For this review, take the finished solid that the model builds, in its own axes (mm). A direction names the side the tool comes from. Coordinates: 2 decimals unless noted, no trailing zeros. Order: outer loops, then holes, each group sorted by start corner. A loop starts at its lowest first (then second) coordinate and runs counter-clockwise, first axis right, second up. Notation, with made-up numbers: (-8, 59) -> (40, 59) arc R17 ccw to (40, 63) -> close; hole circle Ø7 at (45.5, 12). An arc over 180 degrees is marked (long way). Return JSON: item names as keys, results as strings. Group by question number.
Item 1: Take a section at B-B (x = 0). Write out the cut boundary in (y, z), then the cut area to 3 significant figures.
Item 2: For line 1 along Z through (x, y) = (-9.75, -18); line 2 along Y through (x, z) = (0, 36.5); line 3 along Y through (x, z) = (-9.25, -17), list the stretches that pass through material, from the lowest coordinate up.
Item 3: Insertion check: pin 1 (3 mm diameter, centred on x = -8.5, y = -11.5, fed in from -Z); pin 2 (10 mm diameter, centred on y = 8, z = -17, fed in from +X); pin 3 (12 mm diameter, centred on x = -5, y = 11.5, fed in from -Z); pin 4 (5 mm diameter, centred on x = -2.5, z = 23.5, fed in from -Y). Each pin has a flat end and moves straight along its axis. Give the tip position at first contact, or say it passes through.
Item 4: Take a section at A-A (z = 25.5). Write out the cut boundary in (x, y), then the cut area to 3 significant figures.
Item 5: Take a section at D-D (x = 9). Write out the cut boundary in (y, z), then the cut area to 3 significant figures.
Item 6: Machinability: for faces 1 (the flat face through (0, 0, 8)), 2 (the flat face through (12.5, -1, 10)), 3 (the flat face through (-10, -12, 13)), 4 (the flat face through (-6.343, -3, -22)), 5 (the flat face through (-6.5, -12.6, 25.7)), which of the approach directions +Z, -Z, +X, -X, +Y, -Y give a long, thin tool a straight path to every point of the face, cutting with its end or side? Answer none if there is none.
Item 7: Draft analysis for pull direction Z (two halves, no side actions). For faces 6 (the cylindrical face through (-9.542, -30.497, 25.225)), 7 (the flat face through (6.657, -3, -22)), 8 (the cylindrical face through (-9.46, -19.08, 20.62)), state which applies: +Z half, -Z half, draft (parallel to the pull), parting line (faces both ways), or undercut.
Item 8: Take a section at C-C (y = 4.5). Write out the cut boundary in (x, z).
```python
from build123d import *

# Parameters (mm, degrees)
F0_W      = 25
F0_H      = 64
F1_DEPTH  = 6
F2_W      = 25
F2_H      = 6
F3_DEPTH  = 6
F5_DEPTH  = 6
F7_D      = 10
F7_DEPTH  = 13
F7_TIP    = 3.0043030951
F9_D      = 10
F9_DEPTH  = 13
F9_TIP    = 3.0043030951
F11_DEPTH = 12.4


with BuildPart() as f1:
    # F0 (on Front) → F1 (new body)
    with BuildSketch(Plane.XZ):
        Rectangle(F0_W, F0_H)
    extrude(amount=F1_DEPTH)

    # F2 (on face) → F3 (join)
    with BuildSketch(Plane.XY.offset(32)):
        with BuildLine():
            Line((-12.5, 12), (-12.5, 0))
            Line((-12.5, 0), (12.5, 0))
            Line((12.5, 0), (12.5, 12))
            ThreePointArc((12.5, 12), (0, 24.5), (-12.5, 12))
        make_face()
        with Locations((0, -3)):
            Rectangle(F2_W, F2_H)
    extrude(amount=F3_DEPTH)

    # F4 (on face) → F5 (join)
    with BuildSketch(Plane(origin=(-12.5, 0, 0), x_dir=(0, -1, 0), z_dir=(-1, 0, 0))):
        with BuildLine():
            Line((6, 38), (6, 13))
            Line((6, 13), (18, 13))
            ThreePointArc((18, 13), (30.5, 25.5), (18, 38))
            Line((18, 38), (6, 38))
        make_face()
    extrude(amount=-F5_DEPTH)

    # F7
    with Locations(Plane.XY.offset(38)):
        with Locations((0, 12)):
            Hole(F7_D / 2, depth=F7_DEPTH)
            with Locations((0, 0, -(F7_DEPTH + F7_TIP / 2))):  # 118° drill point
                Cone(0, F7_D / 2, F7_TIP, mode=Mode.SUBTRACT)

    # F9
    with Locations(Plane(origin=(-12.5, 0, 0), x_dir=(0, -1, 0), z_dir=(-1, 0, 0))):
        with Locations((18, 25.5)):
            Hole(F9_D / 2, depth=F9_DEPTH)
            with Locations((0, 0, -(F9_DEPTH + F9_TIP / 2))):  # 118° drill point
                Cone(0, F9_D / 2, F9_TIP, mode=Mode.SUBTRACT)

    # F10 (on face) → F11 (cut)
    with BuildSketch(Plane(origin=(0, 0, 0), x_dir=(-1, 0, 0), z_dir=(0, 1, 0))):
        with BuildLine():
            Line((-6.6569247283, -12), (-6.6569247283, -32))
            Line((-6.6569247283, -32), (6.3430752717, -32))
            Line((6.3430752717, -32), (6.3430752717, -12))
            ThreePointArc((6.3430752717, -12), (-0.1569247283, -5.5), (-6.6569247283, -12))
        make_face()
    extrude(amount=-F11_DEPTH, mode=Mode.SUBTRACT)


solid = f1.part
```
Findings below:
{
 "1": {"outline": "(-6, -5.5) -> (0, -5.5) -> (0, 32) -> (7, 32) -> (7, 38) -> (-6, 38) -> close; (17, 32) -> (24.5, 32) -> (24.5, 38) -> (17, 38) -> close", "area": "348 mm2"},
 "2": {"line 1": "z = 13 to 20.5, 30.5 to 38", "line 2": "y = -6 to 7, 17 to 24.5", "line 3": "y = -6 to 0"},
 "3": {"pin 1": "stops at z = 13", "pin 2": "passes through", "pin 3": "stops at z = 32", "pin 4": "stops at y = -6"},
 "4": {"outline": "(-12.5, -30.5) -> (-6.5, -30.5) -> (-6.5, -23) -> (-12.5, -23) -> close; (-12.5, -13) -> (-6.5, -13) -> (-6.5, -6) -> (12.5, -6) -> (12.5, 0) -> (-12.5, 0) -> close", "area": "237 mm2"},
 "5": {"outline": "(-6, -32) -> (0, -32) -> (0, 32) -> (20.67, 32) -> (20.67, 38) -> (-6, 38) -> close", "area": "544 mm2"},
 "6": {"face 1": "-Z, +X, -X, +Y", "face 2": "+Z, -Z, +X, +Y, -Y", "face 3": "-Z, +X, -X, -Y", "face 4": "-Z, +Y, -Y", "face 5": "+Z, -Z, +X, -Y"},
 "7": {"face 6": "parting line", "face 7": "draft", "face 8": "undercut"},
 "8": {"outline": "(-12.5, 32) -> (12.5, 32) -> (12.5, 38) -> (-12.5, 38) -> close"}
}
